Part model, mm, in its own coordinate system. Coordinates: 2 decimals unless noted, no trailing zeros. Loops run counter-clockwise (first coordinate to the right, second up) from the corner with the lowest first, then second, coordinate; pieces in that order, holes last. Notation, with made-up numbers: (35.5, 10) - (50.5, 10) arc R15 cw to (50.5, 33) - close; hole circle Ø1 at (11.25, 83.25). An arc over 180 degrees is marked (long way). Use a Markdown table: item, result. Add a question column.
1. Band-saw the part on A-A, the plane y = 53. Give the cut face in (x, z).
2. Pull direction Y, two halves, no side cores. Call faces 1 (the cylindrical face through (50.69, -52.04, 1.01)), 2 (the cylindrical face through (-60.37, 60.3, 1.01)), 3 (the cylindrical face through (-60.37, -60.3, 1.01)): pulls with the +Y half, pulls with the -Y half, needs draft (parallel to the pull), parting line crosses it, or undercut.
3. Wall check: probe 1 along Y at (x, z) = (53, 0.8). Give the ranges that are in metal, low to high. Write a range as [from, to].
from build123d import *

# Parameters (mm, degrees)
F0_W     = 123.6
F0_H     = 123.6
F1_DEPTH = 2
F2_D     = 5
F2_DEPTH = 4
F3_R     = 5


with BuildPart() as f1:
    # F0 (on Top) → F1 (new body)
    with BuildSketch(Plane.XY):
        Rectangle(F0_W, F0_H)
    extrude(amount=F1_DEPTH)

    # F2
    with Locations(Plane(origin=(0, 0, 0), x_dir=(1, 0, 0), z_dir=(0, 0, -1))):
        with Locations((-53, 53), (53, 53), (-53, -53), (53, -53)):
            Hole(F2_D / 2, depth=F2_DEPTH)

    # F3
    f3_edges = [f1.edges().sort_by_distance(p)[0] for p in [
        (61.8, -61.8, 1),
        (-61.8, -61.8, 1),
        (-61.8, 61.8, 1),
        (61.8, 61.8, 1),
    ]]
    fillet(f3_edges, radius=F3_R)


solid = f1.part
Geometry check:
| question | item | result |
|---|---|---|
| 1 | outline | (-61.8, 0) - (-55.5, 0) - (-55.5, 2) - (-61.8, 2) - close; (-50.5, 0) - (50.5, 0) - (50.5, 2) - (-50.5, 2) - close; (55.5, 0) - (61.8, 0) - (61.8, 2) - (55.5, 2) - close |
| 2 | face 1 | undercut |
| 2 | face 2 | pulls with the +Y half |
| 2 | face 3 | pulls with the -Y half |
| 3 | probe 1 | y = [-61.8, -55.5], [-50.5, 50.5], [55.5, 61.8] |
